Read the model definition and answer for the solid it produces. Units are mm, in the model's axes. Coordinates: 2 decimals unless noted, no trailing zeros. Write each loop counter-clockwise with the first axis right and the second up, starting at its lowest first coordinate (ties: lowest second). Pieces come first, ordered by that corner, then holes. Notation, with made-up numbers: (-22, 83.5) - (27, 83.5) arc R19 cw to (27, 118.5) - close; hole circle Ø7 at (-1.5, 64.5). An arc over 180 degrees is marked (long way). Use a Markdown table: item, result.
from build123d import *

# Parameters (mm, degrees)
SKETCH5_W          = 850.532199311
SKETCH5_H          = 887.458344
CUT_EXTRUDE5_DEPTH = 406.4


with BuildPart() as part:
    # Boss-Extrude1: read off the stored shape, not the designer's step
    # Boss-Extrude1: loft between two sections, ruled curve by curve
    boss_extrude1_from = [
        Edge.make_line((-86.167457674, 1821.517106037, 1121.25455637), (-492.567457674, 1821.517106037, 1451.45455637)),
        Edge.make_line((-492.567457674, 1821.517106037, 1451.45455637), (752.550801769, 2608.917106037, 1451.45455637)),
        Edge.make_line((752.550801769, 2608.917106037, 1451.45455637), (1158.950801769, 2608.917106037, 1121.25455637)),
        Edge.make_line((1158.950801769, 2608.917106037, 1121.25455637), (-86.167457674, 1821.517106037, 1121.25455637)),
    ]
    boss_extrude1_to = [
        Edge.make_line((-89.342457674, 1821.517106037, 1121.25455637), (-495.742457674, 1821.517106037, 1451.45455637)),
        Edge.make_line((-495.742457674, 1821.517106037, 1451.45455637), (749.375801769, 2608.917106037, 1451.45455637)),
        Edge.make_line((749.375801769, 2608.917106037, 1451.45455637), (1155.775801769, 2608.917106037, 1121.25455637)),
        Edge.make_line((1155.775801769, 2608.917106037, 1121.25455637), (-89.342457674, 1821.517106037, 1121.25455637)),
    ]
    boss_extrude1 = Solid(Shell([*[Face.make_surface_from_curves(boss_extrude1_from[k], boss_extrude1_to[k]) for k in range(4)], Face(Wire(boss_extrude1_from)), Face(Wire(boss_extrude1_to))]))
    add(boss_extrude1)

    # Mirror1: Boss-Extrude1 across plane
    add(boss_extrude1.mirror(Plane.XY.offset(1451.45455637)))

    # Sketch5 → Cut-Extrude5 (cut, symmetric)
    with BuildSketch(Plane(origin=(-492.567457674, 0, 0), x_dir=(0, 0, -1), z_dir=(1, 0, 0))):
        with Locations((-1421.298204875, 2221.371463485)):
            Rectangle(SKETCH5_W, SKETCH5_H)
    extrude(amount=CUT_EXTRUDE5_DEPTH, both=True, mode=Mode.SUBTRACT)


solid = part.part
(1) A cutting plane is placed at A-A, the plane z = 1350.5. Write down the section's boundary in (x, y).
Report:
| item | result |
|---|---|
| outline | (-86.17, 1999.94) - (876.8, 2608.92) - (873.63, 2608.92) - (-86.17, 2001.95) - close |
(2) The mould has two halves that part along Z. Classify faces 1 (the flat face through (405.5, 2242.13, 1259.6)), 2 (the flat face through (405.5, 2242.13, 1643.31)), 3 (the flat face through (406.761, 2240.99, 1643.216)): pulls with the +Z half, pulls with the -Z half, needs draft (parallel to the pull), parting line crosses it, or undercut.
Report:
| item | result |
|---|---|
| face 1 | pulls with the -Z half |
| face 2 | pulls with the +Z half |
| face 3 | undercut |
(3) Each of these flat-tipped pins is pushed along its axis until it touches: P1, Ø2, axis at y = 2236, z = 1384, coming from the -X side; P2, Ø1, axis at x = 879.5, z = 1332.5, coming from the +Y side; P3, Ø4, axis at x = 841, z = 1696, coming from the +Y side. Where does it stop, or does it pass through?
Report:
| item | result |
|---|---|
| P1 | stops at x = 240.7 |
| P2 | stops at y = 2599.12 |
| P3 | stops at y = 2478.53 |
(4) A cutting plane is placed at B-B, the plane z = 1607.5. Write down the section's boundary in (x, y), and give its area (3 significant figures).
Report:
| item | result |
|---|---|
| outline | (-86.17, 1957.07) - (944.61, 2608.92) - (941.43, 2608.92) - (-86.17, 1959.07) - close |
| area | 2,070 mm² |
(5) Straight lines are drawn through the part: L1, parallel to Z at x = 730, y = 2426; L2, parallel to Z at x = 731.5, y = 2341.5; L3, parallel to Y at x = 762.5, z = 1277. For each, find the intervals that lie inside material, in ascending order.
Report:
| item | result |
|---|---|
| L1 | z = 1232.18 to 1234.76, 1668.15 to 1670.73 |
| L2 | z = 1122.4 to 1124.98, 1777.93 to 1780.51 |
| L3 | y = 2479.43 to 2481.43 |
